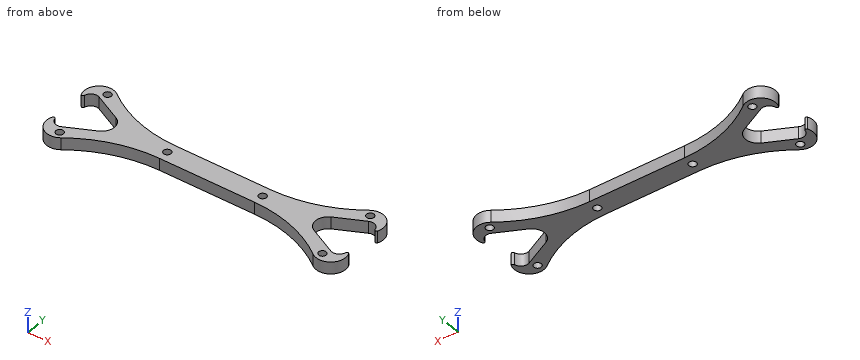
Autodesk Inventor part; units mm, degrees
ref_plane "YZ Plane" through (0, 0, 0) normal (1, 0, 0) x (0, 1, 0)
ref_plane "XZ Plane" through (0, 0, 0) normal (0, 1, 0) x (-1, 0, 0)
ref_plane "XY Plane" through (0, 0, 0) normal (0, 0, 1) x (1, 0, 0)
sketch "Sketch1" plane through (0, 0, 0) normal (0, 0, 1) x (1, 0, 0)
  circle A0 centre (0, 0) radius 1.25
  circle A1 centre (-28.1025, 10.5) radius 1.25
  circle A2 centre (-28.1025, -10.5) radius 1.25
  line L0 (0, 0) -> (-28.1025, 0) construction
  line L1 (-28.1025, 10.5) -> (0, 0) construction
  line L2 (-28.1025, 0) -> (-28.1025, 10.5) construction
  circle A3 centre (0, 0) radius 2.5 construction
  circle A4 centre (-28.1025, 10.5) radius 2.5 construction
  circle A5 centre (-28.1025, -10.5) radius 2.5 construction
  line L3 (0, 0) -> (0, 7) construction
  line L4 (0, 3.5) -> (16, 3.5)
  arc A6 (-26.277, 12.2081) -> (0, 3.5) centre (0, 47.5) ccw
  line L5 (0, -3.5) -> (16, -3.5)
  line L6 (16, 0) -> (16, 5.5221) construction
  circle A7 centre (32, 0) radius 1.25
  circle A8 centre (60.1025, 10.5) radius 1.25
  circle A9 centre (60.1025, -10.5) radius 1.25
  line L7 (32, 0) -> (60.1025, 0) construction
  line L8 (60.1025, 10.5) -> (32, 0) construction
  line L9 (60.1025, 0) -> (60.1025, 10.5) construction
  circle A10 centre (32, 0) radius 2.5 construction
  circle A11 centre (60.1025, 10.5) radius 2.5 construction
  circle A12 centre (60.1025, -10.5) radius 2.5 construction
  line L10 (32, 0) -> (32, 7) construction
  line L11 (32, 3.5) -> (16, 3.5)
  line L12 (32, -3.5) -> (16, -3.5)
  arc A13 (-20.1367, -3.7476) -> (-20.1367, 3.7476) centre (-22, 0) ccw
  arc A14 (-26.277, 12.2081) -> (-33.7448, 6.3389) centre (-29.2155, 8.2614) ccw
  line L13 (-20.1367, 3.7476) -> (-29.2155, 8.2614)
  arc A15 (-29.2155, 8.2614) -> (-32.7919, 6.449) centre (-30.3285, 6.0228) ccw
  arc A16 (-33.7448, 6.3389) -> (-32.7919, 6.449) centre (-33.2846, 6.5343) ccw
  arc A17 (0, -3.5) -> (-26.277, -12.2081) centre (0, -47.5) ccw
  arc A18 (-33.7448, -6.3389) -> (-26.277, -12.2081) centre (-29.2155, -8.2614) ccw
  line L14 (-20.1367, -3.7476) -> (-29.2155, -8.2614)
  arc A19 (-32.7919, -6.449) -> (-29.2155, -8.2614) centre (-30.3285, -6.0228) ccw
  arc A20 (-32.7919, -6.449) -> (-33.7448, -6.3389) centre (-33.2846, -6.5343) ccw
  arc A21 (32, 3.5) -> (58.277, 12.2081) centre (32, 47.5) ccw
  arc A22 (52.1367, 3.7476) -> (52.1367, -3.7476) centre (54, 0) ccw
  arc A23 (65.7448, 6.3389) -> (58.277, 12.2081) centre (61.2155, 8.2614) ccw
  line L15 (52.1367, 3.7476) -> (61.2155, 8.2614)
  arc A24 (64.7919, 6.449) -> (61.2155, 8.2614) centre (62.3285, 6.0228) ccw
  arc A25 (64.7919, 6.449) -> (65.7448, 6.3389) centre (65.2846, 6.5343) ccw
  arc A26 (58.277, -12.2081) -> (32, -3.5) centre (32, -47.5) ccw
  arc A27 (58.277, -12.2081) -> (65.7448, -6.3389) centre (61.2155, -8.2614) ccw
  arc A28 (61.2155, -8.2614) -> (64.7919, -6.449) centre (62.3285, -6.0228) ccw
  line L16 (52.1367, -3.7476) -> (61.2155, -8.2614)
  arc A29 (65.7448, -6.3389) -> (64.7919, -6.449) centre (65.2846, -6.5343) ccw
  dimension "d0" = 2.5
  dimension "d1" = 10.5
  dimension "d2" = 30
  dimension "d3" = 5
  dimension "d22" = 3.5
  dimension "d27" = 16
  dimension "d32" = 0.5
  dimension "d36" = 22
  dimension "d37" = 2.5
  dimension "d38" = 0.5
  dimension "d45" = 88.205
  dimension "d47" = 44
extrude "Extrusion1" add sketch "Sketch1" along normal blind 4
properties part number "legFrame"
CAD build for the part. Positions are in the model's coordinates, mm. Coordinates: 2 decimals unless noted, no trailing zeros. Order: outer loops, then holes, each group sorted by start corner. A loop starts at its lowest first (then second) coordinate and runs counter-clockwise, first axis right, second up. Notation, with made-up numbers: (31, 48.25) - (59, 48.25) arc R33 cw to (59, 85.25) - close; hole circle Ø5 at (70, 89). An arc over 180 degrees is marked (long way). Use a Markdown table: item, result. Add a question column.
(1) Saw through at D-D (x = -6.5). Give the cut face in (y, z), then the cut area to 3 significant figures.
(2) Saw through at B-B (y = -10.5). Give the cut face in (x, z).
(3) Drill centre lines: line 1 along X through (y, z) = (8, 2.7); line 2 along X through (y, z) = (9.5, 3.75); line 3 along Y through (x, z) = (32, 1.7). Where is each one in solid material? Low to high. Write a range as [from, to].
(4) Saw through at A-A (z = 3.2). Count the separate pieces of the cut face and the enclosed holes in it, then the cut area to 3 significant figures.
(5) Flat gauge pin, fed straight in: pin 1 (1 mm diameter, centred on x = 10, z = 2, fed in from +Y). Where does the tip first touch, or does it go through?
(6) Saw through at C-C (x = 36). Give the cut face in (y, z), then the cut area to 3 significant figures.
Solved:
| question | item | result |
|---|---|---|
| 1 | outline | (-3.98, 0) - (3.98, 0) - (3.98, 4) - (-3.98, 4) - close |
| 1 | area | 31.9 mm² |
| 2 | outline | (-33.6, 0) - (-29.35, 0) - (-29.35, 4) - (-33.6, 4) - close; (-26.85, 0) - (-23.81, 0) - (-23.81, 4) - (-26.85, 4) - close; (55.81, 0) - (58.85, 0) - (58.85, 4) - (55.81, 4) - close; (61.35, 0) - (65.6, 0) - (65.6, 4) - (61.35, 4) - close |
| 3 | line 1 | x = [-34.13, -31.86], [-28.69, -19.38], [51.38, 60.69], [63.86, 66.13] |
| 3 | line 2 | x = [-33.98, -28.85], [-27.35, -22.18], [54.18, 59.35], [60.85, 65.98] |
| 3 | line 3 | y = [-3.5, -1.25], [1.25, 3.5] |
| 4 | separate pieces | 1 |
| 4 | enclosed holes | 6 |
| 4 | area | 851 mm² |
| 5 | pin 1 | stops at y = 3.5 |
| 6 | outline | (-3.68, 0) - (3.68, 0) - (3.68, 4) - (-3.68, 4) - close |
| 6 | area | 29.5 mm² |
